Geometry: see drawing. Coordinates: mm, zero at the bounding-box minimum. A direction names the side the tool comes from. Round coordinates to 2 decimals unless told otherwise and drop trailing zeros. Order: outer loops, then holes, each group sorted by start corner. A loop starts at its lowest first (then second) coordinate and runs counter-clockwise, first axis right, second up. Notation, with made-up numbers: (-12.75, 51) - (37.25, 51) arc R14 cw to (37.25, 77) - close; hole circle Ø3 at (24, 35.5). An arc over 180 degrees is marked (long way). Put each result on its own line as item: value. Start each with the question number.
1) Section A-A on x = 1.5. Output: boundary loops of the cut face in (y, z), then the cut area to 3 significant figures.
2) Section B-B on z = 8. Output: boundary loops of the cut face in (x, y).
3) Line query: probe 1 along Y at (x, z) = (8.5, 14.75); probe 2 along Z at (x, y) = (7.75, 14.5); probe 3 along X at (y, z) = (11.5, 8). Output: solid intervals per line, ascending. Write a range as [from, to].
4) Section D-D on y = 3.25. Output: boundary loops of the cut face in (x, z).
5) Mould query, pull axis Y, two halves, no side actions, for the marked faces 4, 5 and 6. Classes: +Y half, -Y half, draft (parallel to the pull), parting line (faces both ways), or undercut.
6) Contact query for flat-ended pins moving along their axis: P1, Ø3, axis at x = 9.5, y = 9, coming from the +Z side; P2, Ø1.5, axis at y = 3.5, z = 13, coming from the +X side; P3, Ø5, axis at x = 12, y = 9, coming from the +Z side. Output: stop coordinate, or through.
7) Section C-C on x = 8. Output: boundary loops of the cut face in (y, z), then the cut area to 4 significant figures.
8) Access query for the marked faces 1, 2 and 3. Directions: +Z, -Z, +X, -X, +Y, -Y. A direction counts if a zero-diameter tool reaches every point of the face in a straight line with its end or side. Return the directions, or none.
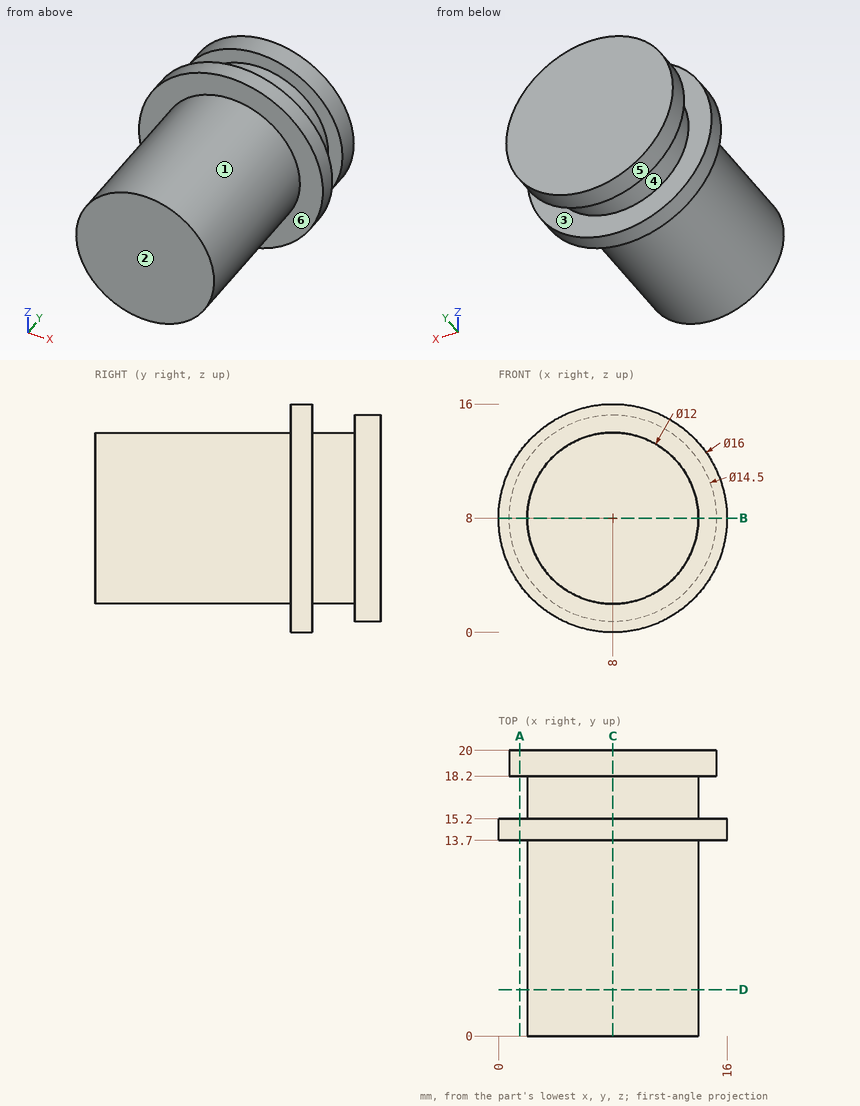
Answer sheet:
1. outline: (13.7, 3.34) - (15.2, 3.34) - (15.2, 12.66) - (13.7, 12.66) - close; (18.2, 4.79) - (20, 4.79) - (20, 11.21) - (18.2, 11.21) - close
1. area: 25.6 mm^2
2. outline: (0, 13.7) - (2, 13.7) - (2, 0) - (14, 0) - (14, 13.7) - (16, 13.7) - (16, 15.2) - (14, 15.2) - (14, 18.2) - (15.25, 18.2) - (15.25, 20) - (0.75, 20) - (0.75, 18.2) - (2, 18.2) - (2, 15.2) - (0, 15.2) - close
3. probe 1: [13.7, 15.2], [18.2, 20]
3. probe 2: [0, 16]
3. probe 3: [2, 14]
4. outline: circle Ø12 at (8, 8)
5. face 4: undercut
5. face 5: draft
5. face 6: -Y half
6. P1: z = 14
6. P2: x = 12.24
6. P3: z = 13.81
7. outline: (0, 2) - (13.7, 2) - (13.7, 0) - (15.2, 0) - (15.2, 2) - (18.2, 2) - (18.2, 0.75) - (20, 0.75) - (20, 15.25) - (18.2, 15.25) - (18.2, 14) - (15.2, 14) - (15.2, 16) - (13.7, 16) - (13.7, 14) - (0, 14) - close
7. area: 250.5 mm^2
8. face 1: -Y
8. face 2: +Z, -Z, +X, -X, -Y
8. face 3: none
